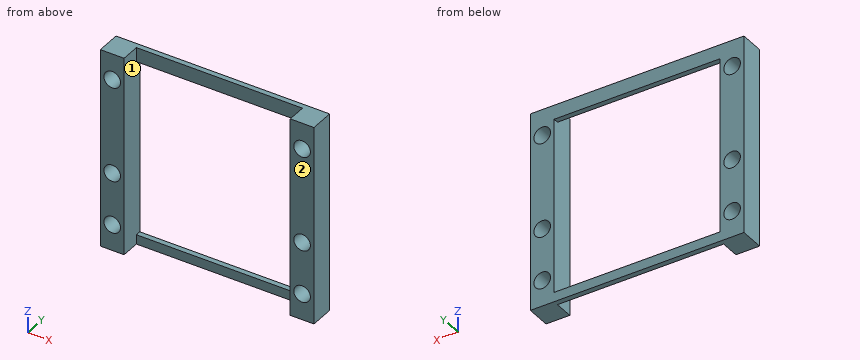
from build123d import *

# Parameters (mm, degrees)
CYLINDER023_R          = 1.75
CYLINDER023_DEPTH      = 44
CYLINDER023_ROLL_ANGLE = 90
CYLINDER024_R          = 1.75
CYLINDER024_DEPTH      = 44
CYLINDER024_ROLL_ANGLE = 90
CYLINDER025_R          = 1.75
CYLINDER025_DEPTH      = 44
CYLINDER025_ROLL_ANGLE = 90
CYLINDER034_R          = 1.75
CYLINDER034_DEPTH      = 44
CYLINDER034_ROLL_ANGLE = 90
CYLINDER035_R          = 1.75
CYLINDER035_DEPTH      = 44
CYLINDER035_ROLL_ANGLE = 90
CYLINDER022_R          = 1.75
CYLINDER022_DEPTH      = 44
CYLINDER022_ROLL_ANGLE = 90
BOX048_W               = 44
BOX048_H               = 1.1
BOX048_DEPTH           = 3
BOX047_W               = 5
BOX047_H               = 5.1
BOX047_DEPTH           = 42
BOX049_W               = 44
BOX049_H               = 1.1
BOX049_DEPTH           = 2
BOX046_W               = 5
BOX046_H               = 5.1
BOX046_DEPTH           = 42


with BuildPart() as cylinder_for_hole_2_motherboard002:
    # Cylinder023 → Cylinder023 (new body)
    with BuildSketch(Plane.XY):
        Circle(CYLINDER023_R)
    extrude(amount=CYLINDER023_DEPTH)


with BuildPart() as cylinder_for_hole_2_motherboard002_1:
    # Cylinder023 roll: moved
    add(cylinder_for_hole_2_motherboard002.part.rotate(Axis((0, 0, 0), (1, 0, 0)), CYLINDER023_ROLL_ANGLE))


with BuildPart() as cylinder_for_hole_2_motherboard002_2:
    # Cylinder023 placement: moved
    add(cylinder_for_hole_2_motherboard002_1.part.moved(Location((20, 6, 17.5))))


with BuildPart() as cylinder_for_hole_9_groovemount_l001:
    # Cylinder024 → Cylinder024 (new body)
    with BuildSketch(Plane.XY):
        Circle(CYLINDER024_R)
    extrude(amount=CYLINDER024_DEPTH)


with BuildPart() as cylinder_for_hole_9_groovemount_l001_1:
    # Cylinder024 roll: moved
    add(cylinder_for_hole_9_groovemount_l001.part.rotate(Axis((0, 0, 0), (1, 0, 0)), CYLINDER024_ROLL_ANGLE))


with BuildPart() as cylinder_for_hole_9_groovemount_l001_2:
    # Cylinder024 placement: moved
    add(cylinder_for_hole_9_groovemount_l001_1.part.moved(Location((-20, 6, -2.5))))


with BuildPart() as cylinder_for_hole_10_groovemount_r001:
    # Cylinder025 → Cylinder025 (new body)
    with BuildSketch(Plane.XY):
        Circle(CYLINDER025_R)
    extrude(amount=CYLINDER025_DEPTH)


with BuildPart() as cylinder_for_hole_10_groovemount_r001_1:
    # Cylinder025 roll: moved
    add(cylinder_for_hole_10_groovemount_r001.part.rotate(Axis((0, 0, 0), (1, 0, 0)), CYLINDER025_ROLL_ANGLE))


with BuildPart() as cylinder_for_hole_10_groovemount_r001_2:
    # Cylinder025 placement: moved
    add(cylinder_for_hole_10_groovemount_r001_1.part.moved(Location((20, 6, -2.5))))


with BuildPart() as cylinder_for_hole_3_motherboard002:
    # Cylinder034 → Cylinder034 (new body)
    with BuildSketch(Plane.XY):
        Circle(CYLINDER034_R)
    extrude(amount=CYLINDER034_DEPTH)


with BuildPart() as cylinder_for_hole_3_motherboard002_1:
    # Cylinder034 roll: moved
    add(cylinder_for_hole_3_motherboard002.part.rotate(Axis((0, 0, 0), (1, 0, 0)), CYLINDER034_ROLL_ANGLE))


with BuildPart() as cylinder_for_hole_3_motherboard002_2:
    # Cylinder034 placement: moved
    add(cylinder_for_hole_3_motherboard002_1.part.moved(Location((-20, 6, -13.5))))


with BuildPart() as cylinder_for_hole_4_motherboard002:
    # Cylinder035 → Cylinder035 (new body)
    with BuildSketch(Plane.XY):
        Circle(CYLINDER035_R)
    extrude(amount=CYLINDER035_DEPTH)


with BuildPart() as cylinder_for_hole_4_motherboard002_1:
    # Cylinder035 roll: moved
    add(cylinder_for_hole_4_motherboard002.part.rotate(Axis((0, 0, 0), (1, 0, 0)), CYLINDER035_ROLL_ANGLE))


with BuildPart() as cylinder_for_hole_4_motherboard002_2:
    # Cylinder035 placement: moved
    add(cylinder_for_hole_4_motherboard002_1.part.moved(Location((20, 6, -13.5))))


with BuildPart() as superstructure_holes:
    # Cylinder022 → Cylinder022 (new body)
    with BuildSketch(Plane.XY):
        Circle(CYLINDER022_R)
    extrude(amount=CYLINDER022_DEPTH)


with BuildPart() as superstructure_holes_1:
    # Cylinder022 roll: moved
    add(superstructure_holes.part.rotate(Axis((0, 0, 0), (1, 0, 0)), CYLINDER022_ROLL_ANGLE))


with BuildPart() as superstructure_holes_2:
    # Cylinder022 placement: moved
    add(superstructure_holes_1.part.moved(Location((-20, 6, 17.5))))

    # Fusion008: union cylinder for hole 2 - Motherboard002, cylinder for hole 9 - Groovemount L001, cylinder for hole 10 - Groovemount R001, cylinder for hole 3 - Motherboard002, cylinder for hole 4 - Motherboard002
    add(cylinder_for_hole_2_motherboard002_2.part)
    add(cylinder_for_hole_9_groovemount_l001_2.part)
    add(cylinder_for_hole_10_groovemount_r001_2.part)
    add(cylinder_for_hole_3_motherboard002_2.part)
    add(cylinder_for_hole_4_motherboard002_2.part)


with BuildPart() as shim_back:
    # Box048 → Box048 (new body)
    with BuildSketch(Plane(origin=(-22, -1, 20), x_dir=(1, 0, 0), z_dir=(0, 0, 1))):
        with Locations((22, 0.55)):
            Rectangle(BOX048_W, BOX048_H)
    extrude(amount=BOX048_DEPTH)


with BuildPart() as shim_l001:
    # Box047 → Box047 (new body)
    with BuildSketch(Plane(origin=(-22.5, -5, -19), x_dir=(1, 0, 0), z_dir=(0, 0, 1))):
        with Locations((2.5, 2.55)):
            Rectangle(BOX047_W, BOX047_H)
    extrude(amount=BOX047_DEPTH)


with BuildPart() as shim_front:
    # Box049 → Box049 (new body)
    with BuildSketch(Plane(origin=(-22, -1, -19), x_dir=(1, 0, 0), z_dir=(0, 0, 1))):
        with Locations((22, 0.55)):
            Rectangle(BOX049_W, BOX049_H)
    extrude(amount=BOX049_DEPTH)


with BuildPart() as superstructure_with_holes:
    # Box046 → Box046 (new body)
    with BuildSketch(Plane(origin=(17.5, -5, -19), x_dir=(1, 0, 0), z_dir=(0, 0, 1))):
        with Locations((2.5, 2.55)):
            Rectangle(BOX046_W, BOX046_H)
    extrude(amount=BOX046_DEPTH)

    # Fusion007: union shim back, shim L001, shim front
    add(shim_back.part)
    add(shim_l001.part)
    add(shim_front.part)

    # Cut007: cut superstructure holes
    add(superstructure_holes_2.part, mode=Mode.SUBTRACT)


solid = superstructure_with_holes.part
Design review of the part built by this model. Coordinates are the model's own, in mm. Face numbers are marked on the shaded views. Give positions to 0.01 mm unless a question says otherwise; leave off trailing zeros. Write each loop counter-clockwise with the first axis right and the second up, starting at its lowest first coordinate (ties: lowest second). Pieces come first, ordered by that corner, then holes. Notation, with made-up numbers: M -6,-11.75 L 40,-11.75 A17 cw 40,19.25 Z; hole C -18.75,64.25 d11. An arc over 180 degrees is marked long. Return JSON: item names as keys, results as strings. Group by question number.
Item 1: Take a section at D-D (x = -8.5). Give the boundary of the cut face in (y, z), plus the area to 3 significant figures.
Item 2: Take a section at C-C (z = -2.5). Give the boundary of the cut face in (x, y), plus the area to 3 significant figures.
Item 3: Clearance check with flat-ended pins moving along their axes: pin 1 Ø4.5 at (x, z) = (20, 17.5) entering from -Y; pin 2 Ø3.5 at (x, z) = (-2, 21.5) entering from -Y. State where each tip first meets the part, or that it passes through.
Item 4: Wall thickness on line 1 along Z through (x, y) = (20, -2); line 2 along X through (y, z) = (-3.75, 17.5); line 3 along X through (y, z) = (-3.8, 15): over which ranges is each line inside the solid? List them lowest first.
Item 5: Take a section at B-B (x = 20). Give the boundary of the cut face in (y, z), plus the area to 3 significant figures.
Item 6: Take a section at A-A (y = -2.7). Give the boundary of the cut face in (x, z), plus the area to 3 significant figures.
Item 7: The part is to be moulded in two halves that separate along X. For the marked faces 1 and 2, say which applies: pulls with the +X half, pulls with the -X half, needs draft (parallel to the pull), parting line crosses it, or undercut.
Return value:
{
 "1": {"outline": "M -1,-19 L 0.1,-19 L 0.1,-17 L -1,-17 Z; M -1,20 L 0.1,20 L 0.1,23 L -1,23 Z", "area": "5.50 mm2"},
 "2": {"outline": "M -22.5,-5 L -21.75,-5 L -21.75,0.1 L -22.5,0.1 Z; M -18.25,-5 L -17.5,-5 L -17.5,0.1 L -18.25,0.1 Z; M 17.5,-5 L 18.25,-5 L 18.25,0.1 L 17.5,0.1 Z; M 21.75,-5 L 22.5,-5 L 22.5,0.1 L 21.75,0.1 Z", "area": "15.3 mm2"},
 "3": {"pin 1": "stops at y = -5", "pin 2": "stops at y = -1"},
 "4": {"line 1": "z = -19 to -15.25, -11.75 to -4.25, -0.75 to 15.75, 19.25 to 23", "line 2": "x = -22.5 to -21.75, -18.25 to -17.5, 17.5 to 18.25, 21.75 to 22.5", "line 3": "x = -22.5 to -17.5, 17.5 to 22.5"},
 "5": {"outline": "M -5,-19 L 0.1,-19 L 0.1,-15.25 L -5,-15.25 Z; M -5,-11.75 L 0.1,-11.75 L 0.1,-4.25 L -5,-4.25 Z; M -5,-0.75 L 0.1,-0.75 L 0.1,15.75 L -5,15.75 Z; M -5,19.25 L 0.1,19.25 L 0.1,23 L -5,23 Z", "area": "161 mm2"},
 "6": {"outline": "M -22.5,-19 L -17.5,-19 L -17.5,23 L -22.5,23 Z; M 17.5,-19 L 22.5,-19 L 22.5,23 L 17.5,23 Z; hole C -20,-13.5 d3.5; hole C -20,-2.5 d3.5; hole C -20,17.5 d3.5; hole C 20,-13.5 d3.5; hole C 20,-2.5 d3.5; hole C 20,17.5 d3.5", "area": "362 mm2"},
 "7": {"face 1": "undercut", "face 2": "needs draft"}
}
